Here's how the part is built. I have some questions about the finished solid (model axes, mm). A direction names the side the tool comes from. Give positions to 0.01 mm unless a question says otherwise; leave off trailing zeros. Loops run counter-clockwise (first coordinate to the right, second up) from the corner with the lowest first, then second, coordinate; pieces in that order, holes last. Notation, with made-up numbers: (55.5, 2) - (86.5, 2) arc R16 ccw to (86.5, 18) - close; hole circle Ø9 at (-22, -21.5). An arc over 180 degrees is marked (long way). Return JSON: item names as keys, results as strings. Group by question number.
(1) I need wall thicknesses on probe 1 along Y at (x, z) = (17.35, -1.45); probe 2 along Z at (x, y) = (18, 1.5); probe 3 along Z at (x, y) = (11, 4.5). Which ranges of each line are inside material? Lowest first, please. Write a range as [from, to].
(2) If we section it at A-A (y = 0.5): Please give me the cut outline in (x, z), then the cut area to 3 significant figures.
(3) If we section it at D-D (x = 21.5): Please give me the cut outline in (y, z), then the cut area to 3 significant figures.
(4) If we mould it in two halves opening along Y, with no side actions, what happens to faces 4 (the cylindrical face through (15.824, 4.481, -3.56)), 5 (the flat face through (18, 8, -2)), 6 (the flat face through (3.711, 1.455, -3.306))? For each: released by +Y, released by -Y, zero draft, split by the parting line, or undercut.
(5) If we section it at B-B (y = 4): Please give me the cut outline in (x, z), then the cut area to 3 significant figures.
(6) On a 3-axis mill with a long thin cutter (end or side, diameter ignored), from which of +Z, -Z, +X, -X, +Y, -Y can I reach the whole of each face in a straight line? I mean faces 1 (the flat face through (19, 3, -0.7)), 2 (the flat face through (9.763, 3.944, -1.872)), 3 (the flat face through (18, 0, -2)). Say none if no direction works.
(7) If we section it at C-C (x = 17.35): Please give me the cut outline in (y, z), then the cut area to 3 significant figures.
(8) For P1, Ø1.5, axis at y = 5.5, z = -1, coming from the -X side; P2, Ø3, axis at x = 17.35, y = 4, coming from the +Z side; P3, Ø4, axis at x = 17.5, y = 2.5, coming from the +Z side, each with a flat end and sliding along its axis, tell me the tip position at first contact or that it passes through.
```python
from build123d import *

# Parameters (mm, degrees)
BOSS_EXTRUDE1_DEPTH       = 8
FILLET1_R                 = 0.1
FILLET2_R                 = 0.5
SKETCH2_R                 = 1.6
CUT_EXTRUDE1_DEPTH        = 36.95822091
REVISION_INDICATION_DEPTH = 0.4


with BuildPart() as part:
    # Sketch1 → Boss-Extrude1 (new body)
    with BuildSketch(Plane(origin=(0, 0, 0), x_dir=(1, 0, 0), z_dir=(0, 1, 0))):
        Polygon((20.35, 0.7), (14.35, 0.7), (0, 0), (-0.117073171, 2.4), (14.35, 4.3), (20.35, 4.3), (34.817073171, 2.4), (34.7, 0), align=None)
        Polygon((20.35, 2.2), (14.35, 2.2), (0.35, 1.2), (14.35, 2.8), (20.35, 2.8), (34.35, 1.2), align=None, mode=Mode.SUBTRACT)
    extrude(amount=BOSS_EXTRUDE1_DEPTH)

    # Fillet1
    fillet1_edges = [part.edges().sort_by_distance(p)[0] for p in [
        (0.35, 4, -1.2),
        (34.35, 4, -1.2),
    ]]
    fillet(fillet1_edges, radius=FILLET1_R)

    # Fillet2
    fillet2_edges = [part.edges().sort_by_distance(p)[0] for p in [
        (-0.117073171, 4, -2.4),
        (34.817073171, 4, -2.4),
        (34.7, 4, 0),
        (0, 4, 0),
    ]]
    fillet(fillet2_edges, radius=FILLET2_R)

    # Sketch2 → Cut-Extrude1 (cut, through all)
    with BuildSketch(Plane(origin=(0, 0, -4.3), x_dir=(-1, 0, 0), z_dir=(0, 0, -1))):
        with Locations((-17.35, 4)):
            Circle(SKETCH2_R)
    extrude(amount=-CUT_EXTRUDE1_DEPTH, mode=Mode.SUBTRACT)

    # Sketch5 → revision indication (add)
    with BuildSketch(Plane(origin=(-0.311839138, 0, -2.374420857), x_dir=(-0.9914858429395939, 0, 0.13021452780071538), z_dir=(-0.13021452780071538, 0, -0.9914858429395939))):
        with BuildLine():
            add(Edge.make_bspline(
                [(-1.75614285, 1.976923077), (-1.720782037, 1.974821832), (-1.651461296, 1.970702586), (-1.551241734, 1.942442049), (-1.460537137, 1.892261337), (-1.379742922, 1.825381725), (-1.313146886, 1.744291021), (-1.261177847, 1.654309873), (-1.233163488, 1.553251269), (-1.229074248, 1.483528859), (-1.226976184, 1.44775641)],
                knots=[0, 0, 0, 0, 1.020151414, 1.999887582, 2.974338812, 3.990962822, 5.007586832, 5.987933904, 6.967670073, 8, 8, 8, 8], degree=3))
            add(Edge.make_bspline(
                [(-1.226976184, 1.44775641), (-1.229145345, 1.412843512), (-1.233422899, 1.343995789), (-1.261113631, 1.243699421), (-1.313542951, 1.153662038), (-1.379283581, 1.071471016), (-1.46055711, 1.004449722), (-1.551456175, 0.954695939), (-1.651226029, 0.924411918), (-1.720742787, 0.920554208), (-1.75614285, 0.918589744)],
                knots=[0, 0, 0, 0, 1.009421747, 1.99056486, 2.972319754, 3.999869655, 5.017953583, 5.993804169, 6.978383603, 8, 8, 8, 8], degree=3))
            add(Edge.make_bspline(
                [(-1.75614285, 0.918589744), (-1.791568422, 0.920483127), (-1.860728417, 0.924179507), (-1.960125864, 0.955317742), (-2.051578507, 1.003983162), (-2.132836213, 1.071595984), (-2.19912744, 1.153239101), (-2.249247777, 1.244319503), (-2.279347047, 1.343708683), (-2.283305588, 1.412786963), (-2.285309517, 1.44775641)],
                knots=[0, 0, 0, 0, 1.022052826, 1.995314843, 2.982371812, 4.00089066, 5.028879526, 6.005146991, 6.990147033, 8, 8, 8, 8], degree=3))
            add(Edge.make_bspline(
                [(-2.285309517, 1.44775641), (-2.283382565, 1.483587428), (-2.279620429, 1.553543092), (-2.249184588, 1.653690044), (-2.199516318, 1.744709926), (-2.132377959, 1.825258007), (-2.051598165, 1.892726399), (-1.960346478, 1.941829667), (-1.860489026, 1.970931558), (-1.791528138, 1.974891267), (-1.75614285, 1.976923077)],
                knots=[0, 0, 0, 0, 1.032775665, 2.016367738, 2.991239715, 4.008302682, 5.025365648, 6.011011707, 6.979408107, 8, 8, 8, 8], degree=3))
        make_face()
        with BuildLine():
            add(Edge.make_bspline(
                [(-4.117040286, 1.976923077), (-4.081679473, 1.974821832), (-4.012358732, 1.970702586), (-3.91213917, 1.942442049), (-3.821434573, 1.892261337), (-3.740640358, 1.825381725), (-3.674044322, 1.744291021), (-3.622075283, 1.654309873), (-3.594060924, 1.553251269), (-3.589971684, 1.483528859), (-3.587873619, 1.44775641)],
                knots=[0, 0, 0, 0, 1.020151414, 1.999887582, 2.974338812, 3.990962822, 5.007586832, 5.987933904, 6.967670073, 8, 8, 8, 8], degree=3))
            add(Edge.make_bspline(
                [(-3.587873619, 1.44775641), (-3.590042781, 1.412843512), (-3.594320335, 1.343995789), (-3.622011067, 1.243699421), (-3.674440387, 1.153662038), (-3.740181017, 1.071471016), (-3.821454546, 1.004449722), (-3.91235361, 0.954695939), (-4.012123464, 0.924411918), (-4.081640223, 0.920554208), (-4.117040286, 0.918589744)],
                knots=[0, 0, 0, 0, 1.009421747, 1.99056486, 2.972319754, 3.999869655, 5.017953583, 5.993804169, 6.978383603, 8, 8, 8, 8], degree=3))
            add(Edge.make_bspline(
                [(-4.117040286, 0.918589744), (-4.152465858, 0.920483127), (-4.221625853, 0.924179507), (-4.3210233, 0.955317742), (-4.412475943, 1.003983162), (-4.493733649, 1.071595984), (-4.560024876, 1.153239101), (-4.610145213, 1.244319503), (-4.640244483, 1.343708683), (-4.644203024, 1.412786963), (-4.646206953, 1.44775641)],
                knots=[0, 0, 0, 0, 1.022052826, 1.995314843, 2.982371812, 4.00089066, 5.028879526, 6.005146991, 6.990147033, 8, 8, 8, 8], degree=3))
            add(Edge.make_bspline(
                [(-4.646206953, 1.44775641), (-4.644280001, 1.483587428), (-4.640517865, 1.553543092), (-4.610082024, 1.653690044), (-4.560413754, 1.744709926), (-4.493275395, 1.825258007), (-4.412495601, 1.892726399), (-4.321243914, 1.941829667), (-4.221386462, 1.970931558), (-4.152425574, 1.974891267), (-4.117040286, 1.976923077)],
                knots=[0, 0, 0, 0, 1.032775665, 2.016367738, 2.991239715, 4.008302682, 5.025365648, 6.011011707, 6.979408107, 8, 8, 8, 8], degree=3))
        make_face()
    extrude(amount=REVISION_INDICATION_DEPTH)


solid = part.part
```
Values:
{
 "1": {"probe 1": "[0, 2.4], [5.6, 8]", "probe 2": "[-4.3, -2.8], [-2.2, -0.7]", "probe 3": "[-3.86, -2.42], [-1.96, -0.54]"},
 "2": {"outline": "(-0.09, -1.94) arc R0.5 ccw to (0.34, -2.46) - (14.35, -4.3) - (20.35, -4.3) - (34.36, -2.46) arc R0.5 ccw to (34.79, -1.94) - (34.72, -0.5) arc R0.5 ccw to (34.2, -0.02) - (20.35, -0.7) - (14.35, -0.7) - (0.5, -0.02) arc R0.5 ccw to (-0.02, -0.5) - close; hole (5.03, -1.73) - (14.35, -2.8) - (20.35, -2.8) - (29.67, -1.73) arc R0.1 ccw to (29.66, -1.54) - (20.35, -2.2) - (14.35, -2.2) - (5.04, -1.54) arc R0.1 ccw to start", "area": "96.9 mm2"},
 "3": {"outline": "(0, -4.15) - (8, -4.15) - (8, -2.67) - (0, -2.67) - close; (0, -2.12) - (8, -2.12) - (8, -0.64) - (0, -0.64) - close", "area": "23.6 mm2"},
 "4": {"face 4": "undercut", "face 5": "released by +Y", "face 6": "zero draft"},
 "5": {"outline": "(-0.09, -1.94) arc R0.5 ccw to (0.34, -2.46) - (14.35, -4.3) - (15.75, -4.3) - (15.75, -2.8) - (14.35, -2.8) - (5.03, -1.73) arc R0.1 cw to (5.04, -1.54) - (14.35, -2.2) - (15.75, -2.2) - (15.75, -0.7) - (14.35, -0.7) - (0.5, -0.02) arc R0.5 ccw to (-0.02, -0.5) - close; (18.95, -4.3) - (20.35, -4.3) - (34.36, -2.46) arc R0.5 ccw to (34.79, -1.94) - (34.72, -0.5) arc R0.5 ccw to (34.2, -0.02) - (20.35, -0.7) - (18.95, -0.7) - (18.95, -2.2) - (20.35, -2.2) - (29.66, -1.54) arc R0.1 cw to (29.67, -1.73) - (20.35, -2.8) - (18.95, -2.8) - close", "area": "87.3 mm2"},
 "6": {"face 1": "+Z, +Y, -Y", "face 2": "+Y, -Y", "face 3": "+Z, -Z, +X, -X, -Y"},
 "7": {"outline": "(0, -4.3) - (2.4, -4.3) - (2.4, -2.8) - (0, -2.8) - close; (0, -2.2) - (2.4, -2.2) - (2.4, -0.7) - (0, -0.7) - close; (5.6, -4.3) - (8, -4.3) - (8, -2.8) - (5.6, -2.8) - close; (5.6, -2.2) - (8, -2.2) - (8, -0.7) - (5.6, -0.7) - close", "area": "14.4 mm2"},
 "8": {"P1": "x = -0.09", "P2": "through", "P3": "z = -0.7"}
}
